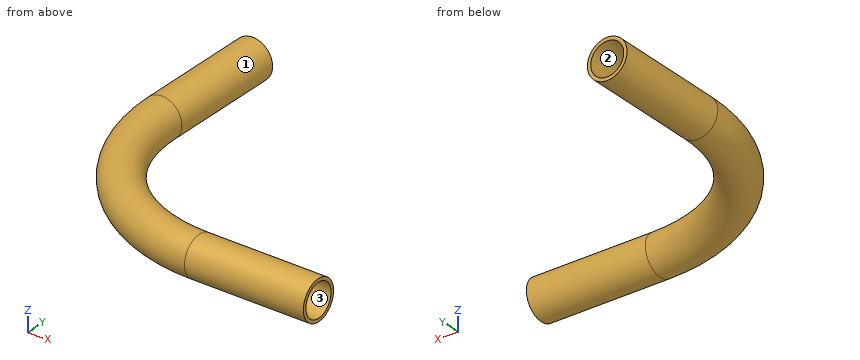
from build123d import *

# Parameters (mm, degrees)
SKETCH1_R                 = 6.35
SKETCH1_R_2               = 5.2832
PIPE_0_5_SCH_40_1_DEPTH   = 38.1
SKETCH1_ON_SEGMENT_2_R    = 6.35
SKETCH1_ON_SEGMENT_2_R_2  = 5.2832
PIPE_0_5_SCH_40_1_2_ANGLE = 90
SKETCH1_ON_SEGMENT_3_R    = 6.35
SKETCH1_ON_SEGMENT_3_R_2  = 5.2832
PIPE_0_5_SCH_40_1_3_DEPTH = 38.1


with BuildPart() as part:
    # Sketch1 → Pipe 0.5 SCH 40(1) (new body)
    with BuildSketch(Plane(origin=(44.524118781, -623.116394341, 354.927728694), x_dir=(1, 0, 0), z_dir=(0, -1, 0))):
        Circle(SKETCH1_R)
        Circle(SKETCH1_R_2, mode=Mode.SUBTRACT)
    extrude(amount=PIPE_0_5_SCH_40_1_DEPTH)


with BuildPart() as body_2:
    # Sketch1 on segment 2 (carried to the start of arc 2) → Pipe 0.5 SCH 40_1 2 (revolve)
    with BuildSketch(Plane(origin=(44.524118781, -661.216394341, 354.927728694), x_dir=(1, 0, 0), z_dir=(0, -1, 0))):
        Circle(SKETCH1_ON_SEGMENT_2_R)
        Circle(SKETCH1_ON_SEGMENT_2_R_2, mode=Mode.SUBTRACT)
    revolve(axis=Axis((95.323978696, -661.216394341, 355.047029303), (-0.002348437, 0, 0.999997242)), revolution_arc=PIPE_0_5_SCH_40_1_2_ANGLE)


with BuildPart() as body_3:
    # Sketch1 on segment 3 (carried to segment 3) → Pipe 0.5 SCH 40_1 3 (new body)
    with BuildSketch(Plane(origin=(95.323978696, -712.016394341, 355.047029303), x_dir=(5.515e-06, 0.999997242, -0.002348431), z_dir=(0.999997242, 0, 0.002348437))):
        Circle(SKETCH1_ON_SEGMENT_3_R)
        Circle(SKETCH1_ON_SEGMENT_3_R_2, mode=Mode.SUBTRACT)
    extrude(amount=PIPE_0_5_SCH_40_1_3_DEPTH)


with BuildPart() as part_1:
    add(part.part)

    # Pipe 0.5 SCH 40(1) as one body: union body 2, body 3
    add(body_2.part)
    add(body_3.part)


solid = part_1.part
Part model, mm, in its own coordinate system. Face numbers are marked on the shaded views. Give positions to 0.01 mm unless a question says otherwise; leave off trailing zeros. Write each loop counter-clockwise with the first axis right and the second up, starting at its lowest first coordinate (ties: lowest second). Pieces come first, ordered by that corner, then holes.
1) Two-plate mould, pull along Z, no slides. Class the marked faces 1, 2 and 3: released by +Z, released by -Z, zero draft, split by the parting line, or undercut.
Resolved:
face 1: split by the parting line
face 2: undercut
face 3: undercut
2) Cut at C-C on y = -641. Write the cut outline in (x, z), then the cut area to 3 significant figures.
Resolved:
outline: circle Ø12.7 at (44.52, 354.93); hole circle Ø10.57 at (44.52, 354.93)
area: 39.0 mm2
3) Pin check, flat tips, straight feed: pin 1 (1 mm diameter, centred on y = -690, z = 360, fed in from +X); pin 2 (4 mm diameter, centred on y = -705.5, z = 352, fed in from +X); pin 3 (1 mm diameter, centred on x = 89.5, z = 359.5, fed in from +Y). Stop position of each tip, or through.
Resolved:
pin 1: stops at x = 59.08
pin 2: stops at x = 133.43
pin 3: stops at y = -706.68
4) Probe L1, parallel to Z at x = 72.5, y = -711; L2, parallel to Y at x = 79, z = 358.25. List the from-to ranges inside material, lowest first.
Resolved:
L1: z = 350.04 to 351.51, 358.49 to 359.96
L2: y = -715.06 to -713.71, -704.9 to -703.52
